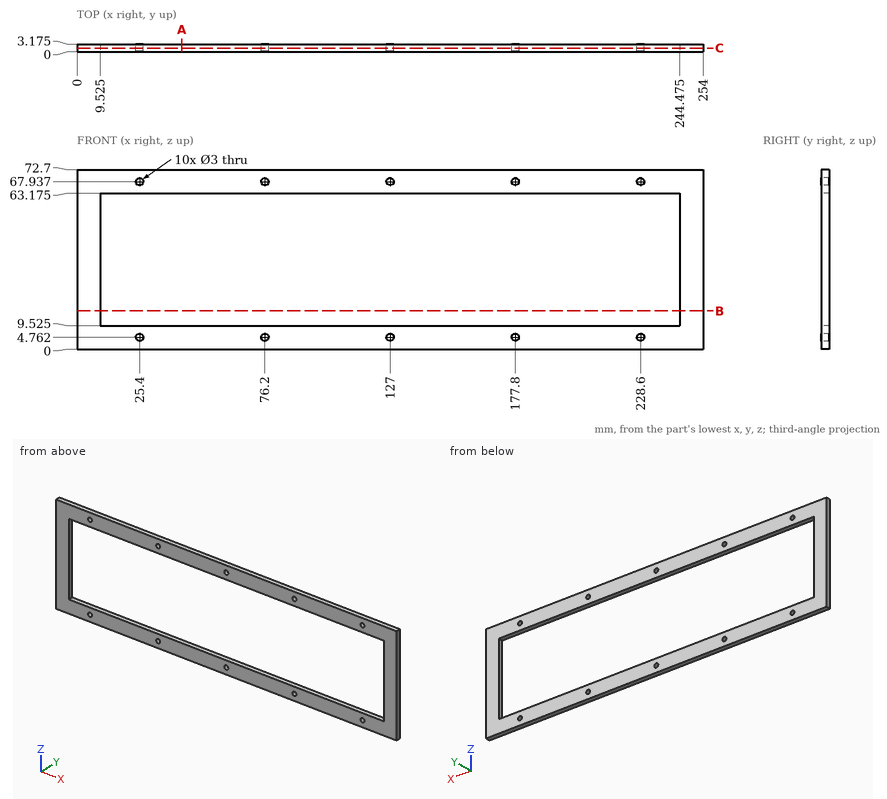
Can you work these out from the drawing? Everything is in mm from the part's minimum corner. Give positions to 0.01 mm unless a question says otherwise; leave off trailing zeros. Loops run counter-clockwise (first coordinate to the right, second up) from the corner with the lowest first, then second, coordinate; pieces in that order, holes last. Notation, with made-up numbers: (0, 34.25) -> (53, 34.25) arc R28 ccw to (53, 54.25) -> close; hole circle Ø10 at (49, 67). An arc over 180 degrees is marked (long way). Write item = value, one per line.
1) Suppose I cut it at C-C on y = 1.55. Give the number of separate pieces and of enclosed holes in the cut face, then the cut area to 3 significant figures.
Check result:
separate_pieces = 1
enclosed_holes = 11
area = 5,790 mm2
2) Suppose I cut it at A-A on x = 42.5. Write out the boundary of the cut face in (y, z) (1 decimal).
Check result:
outline = (0, 0) -> (3.2, 0) -> (3.2, 9.5) -> (0, 9.5) -> close; (0, 63.2) -> (3.2, 63.2) -> (3.2, 72.7) -> (0, 72.7) -> close
3) I need wall thicknesses on L1, parallel to X at y = 1.1, z = 68; L2, parallel to Z at x = 177.5, y = 0.3 (1 decimal); L3, parallel to Z at x = 181, y = 2.05 (1 decimal). Which ranges of each line are inside material? Lowest first, please. Write a range as from..to.
Check result:
L1 = 0..23.9, 26.9..74.7, 77.7..125.5, 128.5..176.3, 179.3..227.1, 230.1..254
L2 = 0..3.3, 6.2..9.5, 63.2..66.5, 69.4..72.7
L3 = 0..9.5, 63.2..72.7
4) Suppose I cut it at B-B on z = 15.5. Write out the boundary of the cut face in (x, y) (1 decimal).
Check result:
outline = (0, 0) -> (9.5, 0) -> (9.5, 3.2) -> (0, 3.2) -> close; (244.5, 0) -> (254, 0) -> (254, 3.2) -> (244.5, 3.2) -> close
5) Will this pin go through, and if not, where does the flat tip stop? pin 1 (2.5 mm diameter, centred on x = 228.6, z = 4.76, fed in from -Y).
Check result:
pin_1 = through
